The drawing under review shows one solid part. Ordinate dimensions are in mm from its lowest x, y, z. Round coordinates to 2 decimals unless told otherwise and drop trailing zeros. Write each loop counter-clockwise with the first axis right and the second up, starting at its lowest first coordinate (ties: lowest second). Pieces come first, ordered by that corner, then holes. Notation, with made-up numbers: (-1.5, -9) -> (46.5, -9) arc R22 ccw to (46.5, 8) -> close; hole circle Ø1 at (24.5, -14.5). An arc over 180 degrees is marked (long way). Write item = value, one per line. Start each with the question number.
Item 1: Add section A-A, the plane y = 12.7. State the section outline as (x, z) points (1 decimal), then the cut area to 3 significant figures.
Item 2: For pin 1 Ø12 at (y, z) = (4, 10.5) entering from -X; pin 2 Ø3 at (y, z) = (15.5, 4.5) entering from +X; pin 3 Ø2 at (x, z) = (6, 13) entering from -Y; pin 4 Ø2 at (x, y) = (22.86, 12.7) entering from +Z, all flat-tipped, find the tip position at first contact; note any pin that passes through.
Item 3: To check wall thickness, follow L1, parallel to Y at x = 8.25, z = 17 (1 decimal); L2, parallel to X at y = 12.5, z = 9.75; L3, parallel to Y at x = 8.75, z = 13 (1 decimal). State the ranges of each line that lie inside material, in increasing order.
Item 4: Add section C-C, the plane z = 14.75. State the section outline as (x, y) points, then the cut area to 3 significant figures.
Item 5: Add section D-D, the plane y = 7.62. State the section outline as (x, z) points (1 decimal), then the cut area to 3 significant figures.
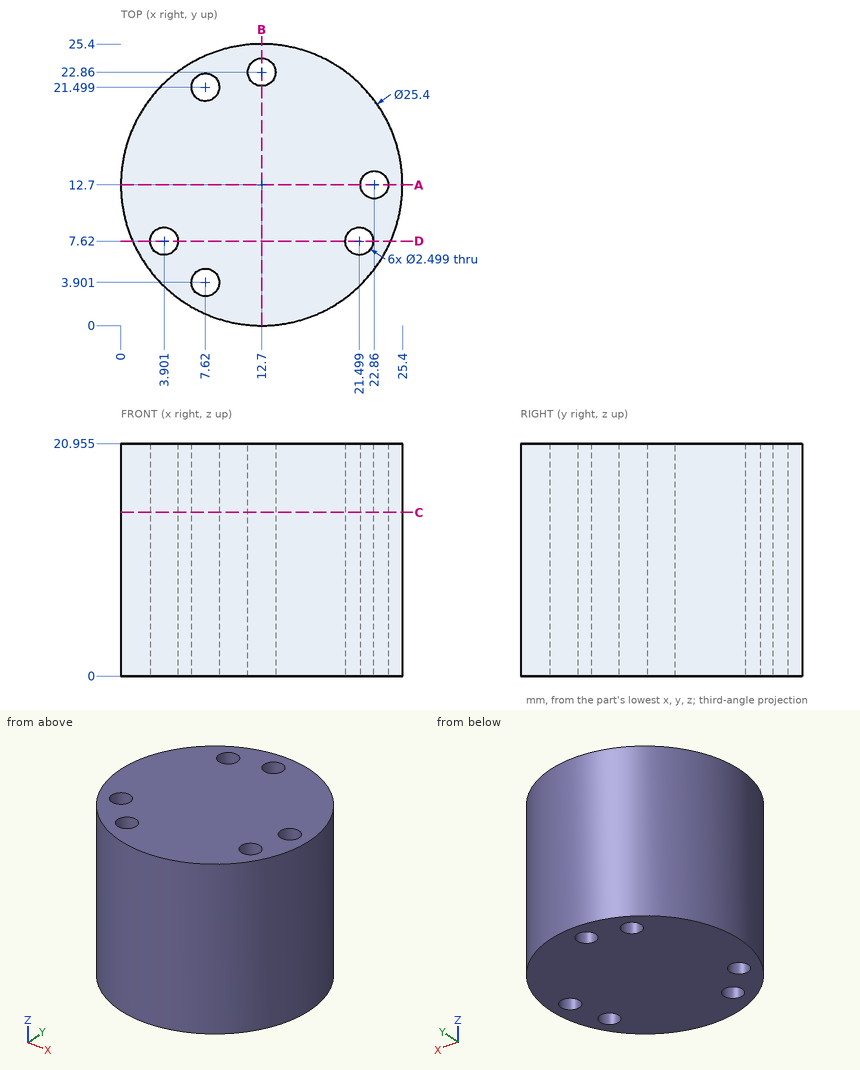
Result set:
q1.outline = (0, 0) -> (21.6, 0) -> (21.6, 21) -> (0, 21) -> close; (24.1, 0) -> (25.4, 0) -> (25.4, 21) -> (24.1, 21) -> close
q1.area = 480 mm²
q2.pin_1 = 0.29
q2.pin_2 = 25.33
q2.pin_3 = 1.35
q2.pin_4 = through
q3.L1 = 0.8 to 2.8, 5 to 20.4, 22.6 to 24.6
q3.L2 = 0 to 21.63, 24.09 to 25.4
q3.L3 = 0.6 to 3.4, 4.4 to 21, 22 to 24.8
q4.outline = circle Ø25.4 at (12.7, 12.7); hole circle Ø2.5 at (3.9, 7.62); hole circle Ø2.5 at (7.62, 3.9); hole circle Ø2.5 at (7.62, 21.5); hole circle Ø2.5 at (12.7, 22.86); hole circle Ø2.5 at (21.5, 7.62); hole circle Ø2.5 at (22.86, 12.7)
q4.area = 477 mm²
q5.outline = (1.1, 0) -> (2.7, 0) -> (2.7, 21) -> (1.1, 21) -> close; (5.2, 0) -> (20.2, 0) -> (20.2, 21) -> (5.2, 21) -> close; (22.7, 0) -> (24.3, 0) -> (24.3, 21) -> (22.7, 21) -> close
q5.area = 383 mm²
